Verification items for the finished model (mm, model axes). Face numbers are marked on the shaded views. A direction names the side the tool comes from. Round coordinates to 2 decimals unless told otherwise and drop trailing zeros. Loops run counter-clockwise (first coordinate to the right, second up) from the corner with the lowest first, then second, coordinate; pieces in that order, holes last. Notation, with made-up numbers: M 38.5,49 L 95.5,49 A11 ccw 95.5,57 Z; hole C -0.5,37.5 d6. An arc over 180 degrees is marked long. Answer as CSV lines item,"result".
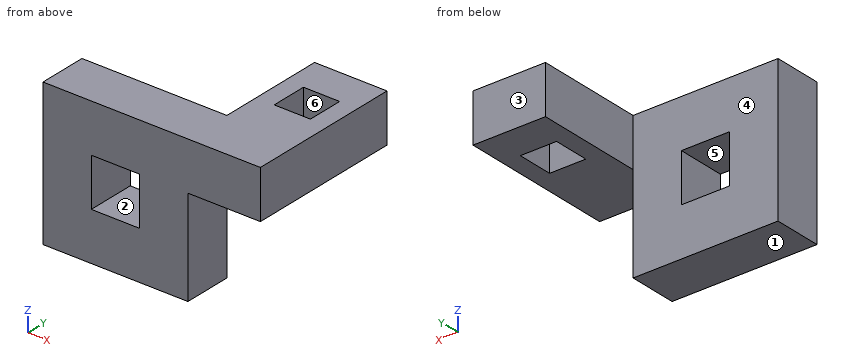
```python
from build123d import *

# Parameters (mm, degrees)
SKETCH1_W           = 60
SKETCH1_H           = 60
SKETCH1_W_2         = 20
SKETCH1_H_2         = 20
BOSS_EXTRUDE1_DEPTH = 20
SKETCH2_W           = 30
SKETCH2_H           = 65
SKETCH2_W_2         = 15
SKETCH2_H_2         = 15
BOSS_EXTRUDE2_DEPTH = 20


with BuildPart() as part:
    # Sketch1 → Boss-Extrude1 (new body)
    with BuildSketch(Plane(origin=(0, 0, 0), x_dir=(1, 0, 0), z_dir=(0, 1, 0))):
        Rectangle(SKETCH1_W, SKETCH1_H)
        Rectangle(SKETCH1_W_2, SKETCH1_H_2, mode=Mode.SUBTRACT)
    extrude(amount=BOSS_EXTRUDE1_DEPTH)

    # Sketch2 → Boss-Extrude2 (add)
    with BuildSketch(Plane.XY.offset(30)):
        with Locations((45, 32.5)):
            Rectangle(SKETCH2_W, SKETCH2_H)
        with Locations((45, 42.5)):
            Rectangle(SKETCH2_W_2, SKETCH2_H_2, mode=Mode.SUBTRACT)
    extrude(amount=-BOSS_EXTRUDE2_DEPTH)


solid = part.part
```
1) Section check B-B (z = 25). Record the cut outline in (x, y).
Here are the results:
outline,"M -30,0 L 60,0 L 60,65 L 30,65 L 30,20 L -30,20 Z; hole M 37.5,35 L 52.5,35 L 52.5,50 L 37.5,50 Z"
2) Section check D-D (z = 3). Record the cut outline in (x, y).
Here are the results:
outline,"M -30,0 L -10,0 L -10,20 L -30,20 Z; M 10,0 L 30,0 L 30,20 L 10,20 Z"
3) Section check A-A (x = 4.5). Record the cut outline in (y, z), plus the area to 3 significant figures.
Here are the results:
outline,"M 0,-30 L 20,-30 L 20,-10 L 0,-10 Z; M 0,10 L 20,10 L 20,30 L 0,30 Z"
area,"800 mm^2"
4) Section check C-C (y = 18.5). Record the cut outline in (x, z).
Here are the results:
outline,"M -30,-30 L 30,-30 L 30,10 L 60,10 L 60,30 L -30,30 Z; hole M -10,-10 L 10,-10 L 10,10 L -10,10 Z"
5) Draft check along Z on the marked faces 1, 2 and 3. Enter one of: +Z half, -Z half, draft (parallel to the pull), parting line (faces both ways), or undercut.
Here are the results:
face 1,"-Z half"
face 2,"undercut"
face 3,"draft"
6) Material ranges on probe 1 along X at (y, z) = (14, -4); probe 2 along Y at (x, z) = (-17, -4.5); probe 3 along Z at (x, y) = (47.5, 31), recorded low to high.
Here are the results:
probe 1,"x = -30 to -10, 10 to 30"
probe 2,"y = 0 to 20"
probe 3,"z = 10 to 30"
7) Go/stop test with flat-tipped pins: pin 1 (10 mm diameter, centred on y = 7, z = -12.5, fed in from +X); pin 2 (16.5 mm diameter, centred on x = 43, z = 16.5, fed in from -Y); pin 3 (1.5 mm diameter, centred on x = 44.5, y = 50, fed in from -Z); pin 4 (6 mm diameter, centred on y = 31.5, z = 22.5, fed in from -X). Record where each tip stops, or that it passes through.
Here are the results:
pin 1,"stops at x = 30"
pin 2,"stops at y = 0"
pin 3,"stops at z = 10"
pin 4,"stops at x = 30"
8) Set-up check for the marked faces 4, 5 and 6: record each of +Z, -Z, +X, -X, +Y, -Y from which the full face is reachable in a straight line by a thin tool's end or side.
Here are the results:
face 4,"+Z, -Z, -X, +Y"
face 5,"+Y, -Y"
face 6,"+Z, -Z"
